from build123d import *

# Parameters (mm, degrees)
ESQUISSE1_W        = 2000
ESQUISSE1_H        = 1000
BOSS_EXTRU_1_DEPTH = 50
ESQUISSE2_W        = 1900
ESQUISSE2_H        = 900
ESQUISSE2_W_2      = 1816
ESQUISSE2_H_2      = 816
BOSS_EXTRU_2_DEPTH = 75
ESQUISSE3_W        = 30
ESQUISSE3_H        = 30
BOSS_EXTRU_3_DEPTH = 1000


with BuildPart() as part:
    # Esquisse1 → Boss.-Extru.1 (new body)
    with BuildSketch(Plane.XY):
        Rectangle(ESQUISSE1_W, ESQUISSE1_H)
    extrude(amount=BOSS_EXTRU_1_DEPTH)

    # Esquisse2 → Boss.-Extru.2 (add)
    with BuildSketch(Plane.XY.offset(50)):
        Rectangle(ESQUISSE2_W, ESQUISSE2_H)
        Rectangle(ESQUISSE2_W_2, ESQUISSE2_H_2, mode=Mode.SUBTRACT)
    extrude(amount=BOSS_EXTRU_2_DEPTH)

    # Esquisse3 → Boss.-Extru.3 (add)
    with BuildSketch(Plane.XY.offset(50)):
        with Locations((-965, 435)):
            Rectangle(ESQUISSE3_W, ESQUISSE3_H)
        with Locations((965, 435)):
            Rectangle(ESQUISSE3_W, ESQUISSE3_H)
        with Locations((965, -435)):
            Rectangle(ESQUISSE3_W, ESQUISSE3_H)
        with Locations((-965, -435)):
            Rectangle(ESQUISSE3_W, ESQUISSE3_H)
    extrude(amount=BOSS_EXTRU_3_DEPTH)


solid = part.part
Design review of the part built by this model. Coordinates are the model's own, in mm. A direction names the side the tool comes from. Round coordinates to 2 decimals unless told otherwise and drop trailing zeros. Write each loop counter-clockwise with the first axis right and the second up, starting at its lowest first coordinate (ties: lowest second). Pieces come first, ordered by that corner, then holes. Notation, with made-up numbers: (89, 1.25) -> (120, 1.25) arc R27 cw to (120, 18.25) -> close; hole circle Ø8 at (-20.75, -40). An arc over 180 degrees is marked (long way). One line per item, written item: value. Start each with the question number.
Q1. Add section D-D (x = 405.5). Give the boundary of the cut face in (y, z).
Q2. Add section A-A (z = 471.5). Give the boundary of the cut face in (x, y).
Q3. Insertion check: P1, Ø24, axis at y = 441, z = 395, coming from the -X side; P2, Ø22.5, axis at y = -12.5, z = 77.5, coming from the -X side; P3, Ø4, axis at x = -136.5, y = 146.5, coming from the +Z side. Each pin has a flat end and moves straight along its axis. Give the tip position at first contact, or say it passes through.
Q4. Add section B-B (y = -198). Give the boundary of the cut face in (x, z).
Q5. Add section C-C (z = 94.5). Give the boundary of the cut face in (x, y).
Q6. To check wall thickness, follow probe 1 along X at (y, z) = (-442, 786); probe 2 along Y at (x, z) = (815.5, 57.5); probe 3 along X at (y, z) = (-180, 58). State the ranges of each line that lie inside material, in increasing order.
Q7. The part is to be moulded in two halves that separate along Y. For faces 5 (the face through (-13, 6, 50)), 6 (the face through (-5, -450, 66)), 7 (the face through (-1000, -7, 25)), say which applies: pulls with the +Y half, pulls with the -Y half, needs draft (parallel to the pull), parting line crosses it, or undercut.
Q8. Tool access review of faces 1 (the face through (-75, -431, 125)), 2 (the face through (-950, -6, 87)), 3 (the face through (-13, -408, 87)), 4 (the face through (950, -6, 87)): name each direction out of +Z, -Z, +X, -X, +Y, -Y from which nothing blocks a thin tool from reaching the whole face with its end or side.
Response:
1. outline: (-500, 0) -> (500, 0) -> (500, 50) -> (450, 50) -> (450, 125) -> (408, 125) -> (408, 50) -> (-408, 50) -> (-408, 125) -> (-450, 125) -> (-450, 50) -> (-500, 50) -> close
2. outline: (-980, -450) -> (-950, -450) -> (-950, -420) -> (-980, -420) -> close; (-980, 420) -> (-950, 420) -> (-950, 450) -> (-980, 450) -> close; (950, -450) -> (980, -450) -> (980, -420) -> (950, -420) -> close; (950, 420) -> (980, 420) -> (980, 450) -> (950, 450) -> close
3. P1: stops at x = -980
3. P2: stops at x = -950
3. P3: stops at z = 50
4. outline: (-1000, 0) -> (1000, 0) -> (1000, 50) -> (950, 50) -> (950, 125) -> (908, 125) -> (908, 50) -> (-908, 50) -> (-908, 125) -> (-950, 125) -> (-950, 50) -> (-1000, 50) -> close
5. outline: (-980, -450) -> (980, -450) -> (980, -420) -> (950, -420) -> (950, 420) -> (980, 420) -> (980, 450) -> (-980, 450) -> (-980, 420) -> (-950, 420) -> (-950, -420) -> (-980, -420) -> close; hole (-908, -408) -> (908, -408) -> (908, 408) -> (-908, 408) -> close
6. probe 1: x = -980 to -950, 950 to 980
6. probe 2: y = -450 to -408, 408 to 450
6. probe 3: x = -950 to -908, 908 to 950
7. face 5: undercut
7. face 6: pulls with the -Y half
7. face 7: needs draft
8. face 1: +Z, +Y, -Y
8. face 2: +Z, -X
8. face 3: +Z
8. face 4: +Z, +X
